```python
from build123d import *

# Parameters (mm, degrees)
ESQUISSE1_R             = 11
ESQUISSE1_R_2           = 4
BOSS_EXTRU_1_DEPTH      = 7
ESQUISSE2_R             = 8.959660805
ESQUISSE2_R_2           = 5.876621398
ENL_V_MAT_EXTRU_1_DEPTH = 0.5


with BuildPart() as part:
    # Esquisse1 → Boss.-Extru.1 (new body)
    with BuildSketch(Plane(origin=(0, 0, 0), x_dir=(1, 0, 0), z_dir=(0, 1, 0))):
        Circle(ESQUISSE1_R)
        Circle(ESQUISSE1_R_2, mode=Mode.SUBTRACT)
    extrude(amount=BOSS_EXTRU_1_DEPTH)

    # Esquisse2 → Enlèv. mat.-Extru.1 (cut)
    with BuildSketch(Plane(origin=(0, 7, 0), x_dir=(1, 0, 0), z_dir=(0, 1, 0))):
        Circle(ESQUISSE2_R)
        Circle(ESQUISSE2_R_2, mode=Mode.SUBTRACT)
    enl_v_mat_extru_1 = extrude(amount=-ENL_V_MAT_EXTRU_1_DEPTH, mode=Mode.SUBTRACT)

    # Symétrie1: Enlèv. mat.-Extru.1 across plane
    add(enl_v_mat_extru_1.mirror(Plane.ZX.offset(3.5)), mode=Mode.SUBTRACT)


solid = part.part
```
Input: part model. Units: mm. Frame: model coordinates. A direction names the side the tool comes from. Round coordinates to 2 decimals unless told otherwise and drop trailing zeros. Write each loop counter-clockwise with the first axis right and the second up, starting at its lowest first coordinate (ties: lowest second). Pieces come first, ordered by that corner, then holes. Notation, with made-up numbers: M 75,-12.75 L 115,-12.75 A6 ccw 115,-4.75 Z; hole C 18,-15 d11. An arc over 180 degrees is marked long. Write each question's results on one line, items separated by ' | '.
Q1. Line query: line 1 along Z through (x, y) = (0, 6.75); line 2 along Z through (x, y) = (0, 5). Output: solid intervals per line, ascending.
Results:
line 1: z = -11 to -8.96, -5.88 to -4, 4 to 5.88, 8.96 to 11 | line 2: z = -11 to -4, 4 to 11
Q2. Pin query (flat end, axial travel): P1, Ø1, axis at x = 4.5, y = 2.5, coming from the +Z side; P2, Ø1.5, axis at x = 7.5, y = 4, coming from the -Z side; P3, Ø1, axis at y = 5.5, z = -2, coming from the +X side. Return the tip coordinate at first contact, or that it passes through.
Results:
P1: stops at z = 10.25 | P2: stops at z = -8.69 | P3: stops at x = 10.9
Q3. Draft query along Z for faces 4 (the face through (-1.274, 6.754, 5.737)), 5 (the face through (2, 0, 9)), 6 (the face through (-2.38, 3.45, 10.74)). Return one class per face: released by +Z, released by -Z, zero draft, split by the parting line, or undercut.
Results:
face 4: undercut | face 5: zero draft | face 6: split by the parting line
Q4. Section query D-D (y = 4.25). Return loops of the section in (x, z), and give its area (3 significant figures).
Results:
outline: C 0,0 d22; hole C 0,0 d8 | area: 330 mm^2
Q5. Access query for faces 1 (the face through (2, 7, 9)), 2 (the face through (4.817, 0.246, -7.555)), 3 (the face through (2, 6.5, 6)). Directions: +Z, -Z, +X, -X, +Y, -Y. A direction counts if a zero-diameter tool reaches every point of the face in a straight line with its end or side. Return the directions, or none.
Results:
face 1: +Z, -Z, +X, -X, +Y | face 2: -Y | face 3: +Y
Q6. Section query C-C (z = 6.5). Return loops of the section in (x, y), and give its area (3 significant figures).
Results:
outline: M -8.87,0 L -6.17,0 L -6.17,0.5 L 6.17,0.5 L 6.17,0 L 8.87,0 L 8.87,7 L 6.17,7 L 6.17,6.5 L -6.17,6.5 L -6.17,7 L -8.87,7 Z | area: 112 mm^2
Q7. Section query A-A (x = 0). Return loops of the section in (y, z).
Results:
outline: M 0,-11 L 7,-11 L 7,-8.96 L 6.5,-8.96 L 6.5,-5.88 L 7,-5.88 L 7,-4 L 0,-4 L 0,-5.88 L 0.5,-5.88 L 0.5,-8.96 L 0,-8.96 Z; M 0,4 L 7,4 L 7,5.88 L 6.5,5.88 L 6.5,8.96 L 7,8.96 L 7,11 L 0,11 L 0,8.96 L 0.5,8.96 L 0.5,5.88 L 0,5.88 Z
Q8. Section query B-B (z = 0). Return loops of the section in (x, y).
Results:
outline: M -11,0 L -8.96,0 L -8.96,0.5 L -5.88,0.5 L -5.88,0 L -4,0 L -4,7 L -5.88,7 L -5.88,6.5 L -8.96,6.5 L -8.96,7 L -11,7 Z; M 4,0 L 5.88,0 L 5.88,0.5 L 8.96,0.5 L 8.96,0 L 11,0 L 11,7 L 8.96,7 L 8.96,6.5 L 5.88,6.5 L 5.88,7 L 4,7 Z
